from build123d import *

# Parameters (mm, degrees)
BOX017_W          = 4
BOX017_H          = 16
BOX017_DEPTH      = 10
CYLINDER022_R     = 2
CYLINDER022_DEPTH = 10
BOX016_W          = 8.2
BOX016_H          = 15
BOX016_DEPTH      = 10
BOX015_W          = 8.52
BOX015_H          = 15
BOX015_DEPTH      = 10
BOX014_W          = 44
BOX014_H          = 15
BOX014_DEPTH      = 2.6
BOX013_W          = 44
BOX013_H          = 30
BOX013_DEPTH      = 5


with BuildPart() as cube017:
    # Box017 → Box017 (new body)
    with BuildSketch(Plane(origin=(20, -8, 0), x_dir=(1, 0, 0), z_dir=(0, 0, 1))):
        with Locations((2, 8)):
            Rectangle(BOX017_W, BOX017_H)
    extrude(amount=BOX017_DEPTH)


with BuildPart() as fusion022:
    # Cylinder022 → Cylinder022 (new body)
    with BuildSketch(Plane(origin=(22, 8, 0), x_dir=(1, 0, 0), z_dir=(0, 0, 1))):
        Circle(CYLINDER022_R)
    extrude(amount=CYLINDER022_DEPTH)

    # Fusion022: union Cube017
    add(cube017.part)


with BuildPart() as cube016:
    # Box016 → Box016 (new body)
    with BuildSketch(Plane(origin=(35.8, 0, 0), x_dir=(1, 0, 0), z_dir=(0, 0, 1))):
        with Locations((4.1, 7.5)):
            Rectangle(BOX016_W, BOX016_H)
    extrude(amount=BOX016_DEPTH)


with BuildPart() as cube015:
    # Box015 → Box015 (new body)
    with BuildSketch(Plane.XY):
        with Locations((4.26, 7.5)):
            Rectangle(BOX015_W, BOX015_H)
    extrude(amount=BOX015_DEPTH)


with BuildPart() as cube014:
    # Box014 → Box014 (new body)
    with BuildSketch(Plane.XY):
        with Locations((22, 7.5)):
            Rectangle(BOX014_W, BOX014_H)
    extrude(amount=BOX014_DEPTH)


with BuildPart() as exterior_part1:
    # Box013 → Box013 (new body)
    with BuildSketch(Plane.XY):
        with Locations((22, 15)):
            Rectangle(BOX013_W, BOX013_H)
    extrude(amount=BOX013_DEPTH)

    # Cut007002002: cut Cube014
    add(cube014.part, mode=Mode.SUBTRACT)

    # Cut007002003: cut Cube015
    add(cube015.part, mode=Mode.SUBTRACT)

    # Cut007002004: cut Cube016
    add(cube016.part, mode=Mode.SUBTRACT)

    # Cut007002005: cut Fusion022
    add(fusion022.part, mode=Mode.SUBTRACT)


with BuildPart() as exterior_part1_1:
    # Cut007002005 placement: moved
    add(exterior_part1.part.moved(Location((0, 21, 0))))


solid = exterior_part1_1.part
Model file for the job. Use its own axes, mm. A direction names the side the tool comes from. Round coordinates to 2 decimals unless told otherwise and drop trailing zeros. Order: outer loops, then holes, each group sorted by start corner. A loop starts at its lowest first (then second) coordinate and runs counter-clockwise, first axis right, second up. Notation, with made-up numbers: M -0.5,-25 L 48.5,-25 A31 cw 48.5,3 Z; hole C 21,32.25 d10. An arc over 180 degrees is marked long. Write each question's results on one line, items separated by ' | '. Start each with the question number.
(1) Which spindle directions (+Z, -Z, +X, -X, +Y, -Y) get a long thin tool onto all of the face, cutting with end or side? Do faces 4 (the face through (22, 51, 2)), 5 (the face through (25, 29, 2.6)), 6 (the face through (24, 25, 4)), 7 (the face through (0, 43, 2)), 8 (the face through (35.8, 28, 4)). Say none if no direction does.
(2) Probe probe 1 along X at (y, z) = (25.75, 3.45); probe 2 along Z at (x, y) = (13, 30.75); probe 3 along Y at (x, z) = (36, 4.5). List the from-to ranges inside material, lowest first. Write a range as from..to.
(3) Saw through at A-A, the plane y = 27. Give the cut face in (x, z).
(4) Saw through at C-C, the plane z = 0.5. Give the cut face in (x, y).
(5) Saw through at D-D, the plane x = 37. Give the cut face in (y, z).
(6) Two-plate mould, pull along X, no slides. Class faces 1 (the face through (20, 25, 4)), 2 (the face through (22, 40, 5)), 3 (the face through (8.52, 28, 4)): pulls with the +X half, pulls with the -X half, needs draft (parallel to the pull), parting line crosses it, or undercut.
(7) Saw through at B-B, the plane x = 22. Give the cut face in (y, z), then the cut area to 3 significant figures.
(8) Drop flat-ended pins along their axis: pin 1 (2.5 mm diameter, centred on y = 29.5, z = 3.5, fed in from -X); pin 2 (3 mm diameter, centred on x = 8.5, z = 1, fed in from -Y); pin 3 (2.5 mm diameter, centred on y = 29, z = 4, fed in from +X). Give the stop position or say it passes through.
Established:
1) face 4: +Z, -Z, +X, -X, +Y | face 5: -Z, +X, -X, -Y | face 6: +Z, -Z, -Y | face 7: +Z, -Z, -X, +Y, -Y | face 8: +Z, -Z, +X, -Y
2) probe 1: x = 8.52..20, 24..35.8 | probe 2: z = 2.6..5 | probe 3: y = 36..51
3) outline: M 8.52,2.6 L 20,2.6 L 20,5 L 8.52,5 Z; M 24,2.6 L 35.8,2.6 L 35.8,5 L 24,5 Z
4) outline: M 0,36 L 44,36 L 44,51 L 0,51 Z
5) outline: M 36,0 L 51,0 L 51,5 L 36,5 Z
6) face 1: undercut | face 2: needs draft | face 3: pulls with the -X half
7) outline: M 31,2.6 L 36,2.6 L 36,0 L 51,0 L 51,5 L 31,5 Z | area: 87.0 mm^2
8) pin 1: stops at x = 8.52 | pin 2: stops at y = 36 | pin 3: stops at x = 35.8
